Could you check a few things on this model? Use its own coordinates, in mm. Face numbers are marked on the shaded views. A direction names the side the tool comes from. Give positions to 0.01 mm unless a question says otherwise; leave off trailing zeros. Loops run counter-clockwise (first coordinate to the right, second up) from the corner with the lowest first, then second, coordinate; pieces in that order, holes last. Notation, with made-up numbers: (15, 54) - (36, 54) arc R13 cw to (36, 67) - close; hole circle Ø10 at (10.25, -13). An arc over 180 degrees is marked (long way). Write each question's results on one line, items separated by ' | '. Start each with the question number.
(1) Suppose I cut it at C-C (x = 20). Please give me the cut outline in (y, z), and give its area (3 significant figures).
(2) Suppose I cut it at D-D (x = -16.5). Please give me the cut outline in (y, z), and give its area (3 significant figures).
(3) For pin 1 (5 mm diameter, centred on x = -11.5, z = -4, fed in from -Y); pin 2 (6 mm diameter, centred on x = -0.5, y = -4, fed in from +Z); pin 3 (1.5 mm diameter, centred on x = 12, z = 3.5, fed in from -Y); pin 4 (5 mm diameter, centred on x = -5, y = -0.5, fed in from +Z), each with a flat end and sliding along its axis, tell me the tip position at first contact or that it passes through.
(4) I need wall thicknesses on line 1 (Y direction, x = -13.5, z = 0.25); line 2 (X direction, y = -4.25, z = -2); line 3 (Y direction, x = -20, z = -3.25). Which ranges of each line are inside material? Lowest first, please.
(5) Suppose I cut it at A-A (y = 0). Please give me the cut outline in (x, z), and give its area (4 significant figures).
(6) On a 3-axis mill with a long thin cutter (end or side, diameter ignored), from which of +Z, -Z, +X, -X, +Y, -Y can I reach the whole of each face in a straight line? I mean the marked faces 1, 2 and 3. Say none if no direction works.
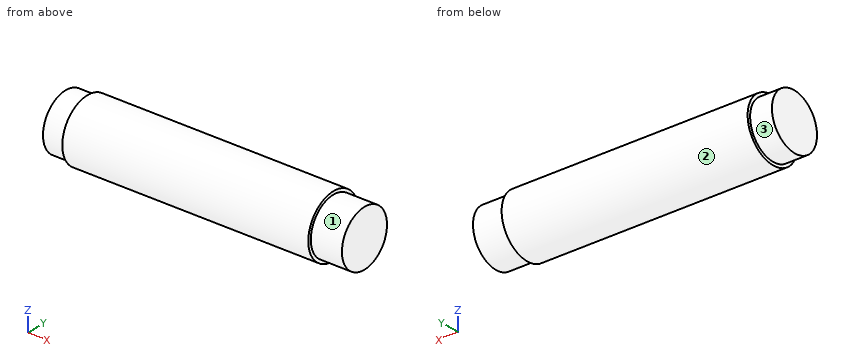
from build123d import *

# Parameters (mm, degrees)
SKETCH1_R                = 5
BOSS_EXTRUDE1_DEPTH      = 19
BOSS_EXTRUDE1_DEPTH_BACK = 20.5
SKETCH2_R                = 4.5
BOSS_EXTRUDE2_DEPTH      = 5


with BuildPart() as part:
    # Sketch1 → Boss-Extrude1 (new body, two sides)
    with BuildSketch(Plane(origin=(0, 0, 0), x_dir=(0, 0, -1), z_dir=(1, 0, 0))) as boss_extrude1_sk:
        Circle(SKETCH1_R)
    extrude(amount=BOSS_EXTRUDE1_DEPTH)
    extrude(boss_extrude1_sk.sketch, amount=-BOSS_EXTRUDE1_DEPTH_BACK)

    # Sketch2 → Boss-Extrude2 (add)
    with BuildSketch(Plane(origin=(19, 0, 0), x_dir=(0, 0, -1), z_dir=(1, 0, 0))):
        Circle(SKETCH2_R)
    boss_extrude2 = extrude(amount=BOSS_EXTRUDE2_DEPTH)

    # Mirror1: Boss-Extrude2 across plane
    add(boss_extrude2.mirror(Plane(origin=(0, 0, 0), x_dir=(0, 0, 1), z_dir=(1, 0, 0))))


solid = part.part
Output values:
1) outline: circle Ø9 at (0, 0) | area: 63.6 mm2
2) outline: circle Ø10 at (0, 0) | area: 78.5 mm2
3) pin 1: y = -4.77 | pin 2: z = 4.9 | pin 3: y = -4.18 | pin 4: z = 5
4) line 1: -4.99 to 4.99 | line 2: -20.5 to 19 | line 3: -3.8 to 3.8
5) outline: (-24, -4.5) - (-20.5, -4.5) - (-20.5, -5) - (19, -5) - (19, -4.5) - (24, -4.5) - (24, 4.5) - (19, 4.5) - (19, 5) - (-20.5, 5) - (-20.5, 4.5) - (-24, 4.5) - close | area: 471.5 mm2
6) face 1: +X | face 2: +X, -X | face 3: -X
